The drawing under review shows one solid part. Ordinate dimensions are in mm from its lowest x, y, z. Coordinates: 2 decimals unless noted, no trailing zeros. Loops run counter-clockwise (first coordinate to the right, second up) from the corner with the lowest first, then second, coordinate; pieces in that order, holes last. Notation, with made-up numbers: M 24.25,47 L 40.25,47 A19 cw 40.25,78 Z; hole C 15.5,-12 d9. An arc over 180 degrees is marked long. Return JSON: item names as keys, results as strings.
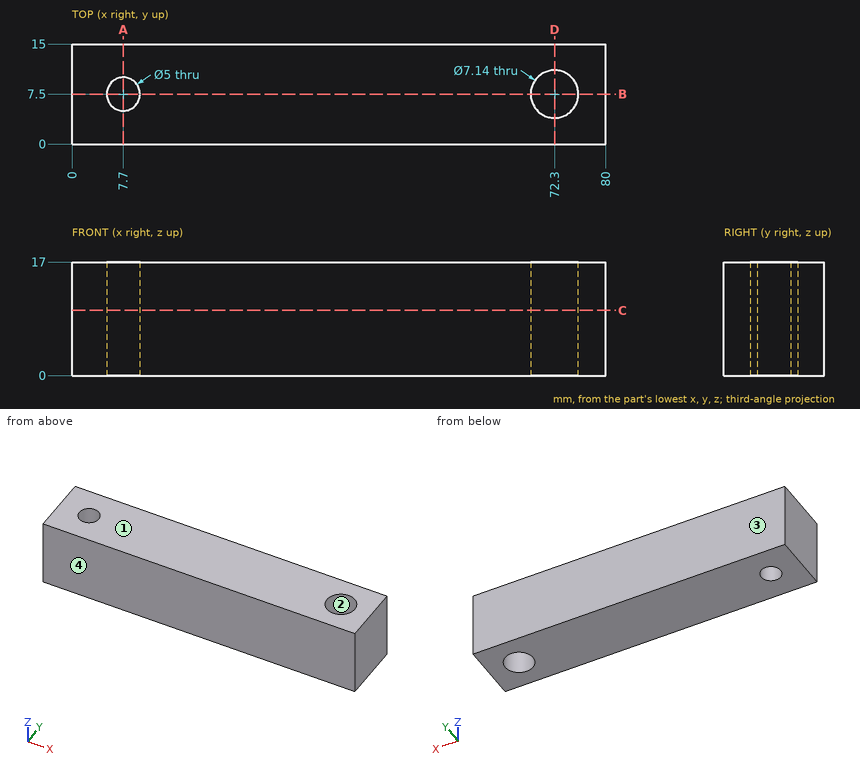
1. Add section A-A on x = 7.7. Give the boundary of the cut face in (y, z), plus the area to 3 significant figures.
Check values:
{"outline": "M 0,0 L 5,0 L 5,17 L 0,17 Z; M 10,0 L 15,0 L 15,17 L 10,17 Z", "area": "170 mm²"}
2. The part is to be moulded in two halves that separate along Y. For the marked faces 1, 2, 3 and 4, say which applies: released by +Y, released by -Y, zero draft, split by the parting line, or undercut.
Check values:
{"face 1": "zero draft", "face 2": "undercut", "face 3": "released by +Y", "face 4": "released by -Y"}
3. Add section D-D on x = 72.3. Give the boundary of the cut face in (y, z), plus the area to 3 significant figures.
Check values:
{"outline": "M 0,0 L 3.93,0 L 3.93,17 L 0,17 Z; M 11.07,0 L 15,0 L 15,17 L 11.07,17 Z", "area": "134 mm²"}
4. Add section B-B on y = 7.5. Give the boundary of the cut face in (x, z), plus the area to 3 significant figures.
Check values:
{"outline": "M 0,0 L 5.2,0 L 5.2,17 L 0,17 Z; M 10.2,0 L 68.73,0 L 68.73,17 L 10.2,17 Z; M 75.87,0 L 80,0 L 80,17 L 75.87,17 Z", "area": "1,150 mm²"}
5. To check wall thickness, follow line 1 (Y direction, x = 7.7, z = 10.5); line 2 (X direction, y = 8.5, z = 7); line 3 (Y direction, x = 72.3, z = 12.5). State the ranges of each line that lie inside material, in increasing order.
Check values:
{"line 1": "0 to 5, 10 to 15", "line 2": "0 to 5.41, 9.99 to 68.87, 75.73 to 80", "line 3": "0 to 3.93, 11.07 to 15"}
6. Insertion check: pin 1 Ø4.5 at (x, y) = (7.7, 7.5) entering from +Z. The pin has a flat end and moves straight along its axis. Give the tip position at first contact, or say it passes through.
Check values:
{"pin 1": "through"}
7. Add section C-C on z = 9.75. Give the boundary of the cut face in (x, y), plus the area to 3 significant figures.
Check values:
{"outline": "M 0,0 L 80,0 L 80,15 L 0,15 Z; hole C 7.7,7.5 d5; hole C 72.3,7.5 d7.14", "area": "1,140 mm²"}
